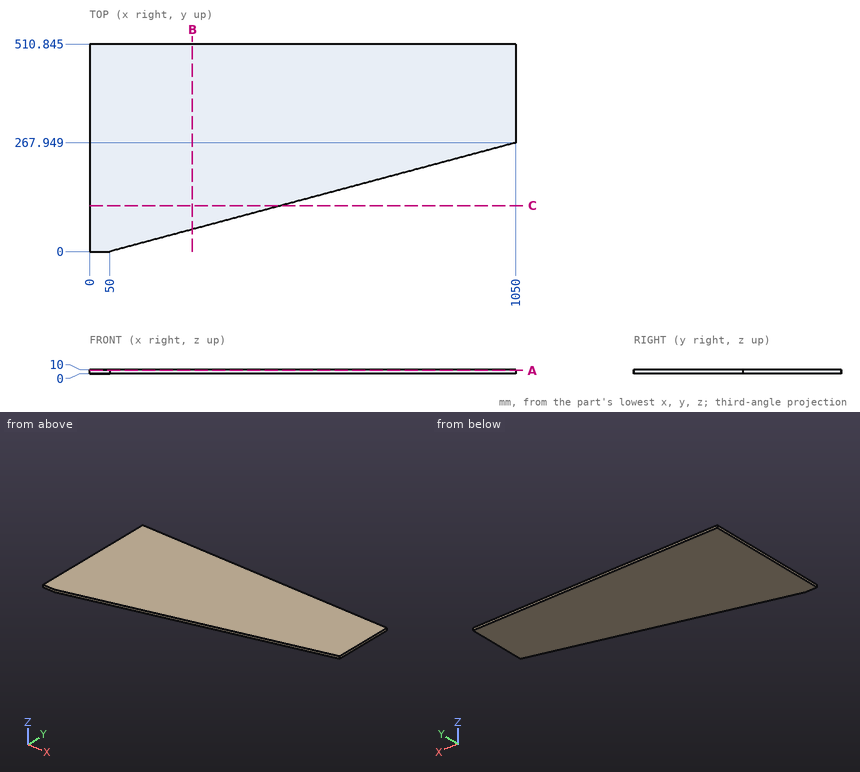
Input: dimensioned drawing with shaded views. Units: mm. Origin: part minimum x, y, z. Round coordinates to 2 decimals unless told otherwise and drop trailing zeros. Loops run counter-clockwise (first coordinate to the right, second up) from the corner with the lowest first, then second, coordinate; pieces in that order, holes last. Notation, with made-up numbers: M 9.25,-27.5 L 40.25,-27.5 A25 cw 40.25,4.5 Z; hole C 23.25,-40 d1. An arc over 180 degrees is marked long. Return JSON: item names as keys, results as strings. Group by question number.
1. Material intervals for line 1 along Y through (x, z) = (462, 3) (1 decimal); line 2 along Y through (x, z) = (240, 6) (1 decimal), sorted ascending. Write a range as from..to.
2. Pin query (flat end, axial travel): pin 1 (6 mm diameter, centred on x = 628, z = 2, fed in from -Y). Return the tip coordinate at first contact, or that it passes through.
3. Section query B-B on x = 253. Output: boundary loops of the cut face in (y, z) (1 decimal).
4. Section query C-C on y = 113. Output: boundary loops of the cut face in (x, z).
5. Section query A-A on z = 8. Output: boundary loops of the cut face in (x, y) (1 decimal).
Checks:
{
 "1": {"line 1": "y = 110.4..510.8", "line 2": "y = 50.9..510.8"},
 "2": {"pin 1": "stops at y = 154.07"},
 "3": {"outline": "M 54.4,0 L 510.8,0 L 510.8,10 L 54.4,10 Z"},
 "4": {"outline": "M 0,0 L 471.72,0 L 471.72,10 L 0,10 Z"},
 "5": {"outline": "M 0,0 L 50,0 L 1050,267.9 L 1050,510.8 L 0,510.8 Z"}
}
